Print and shaded views of the part. All mm, measured from the part's lowest x, y and z. A direction names the side the tool comes from. Coordinates: 2 decimals unless noted, no trailing zeros. Write item = value, one per line.
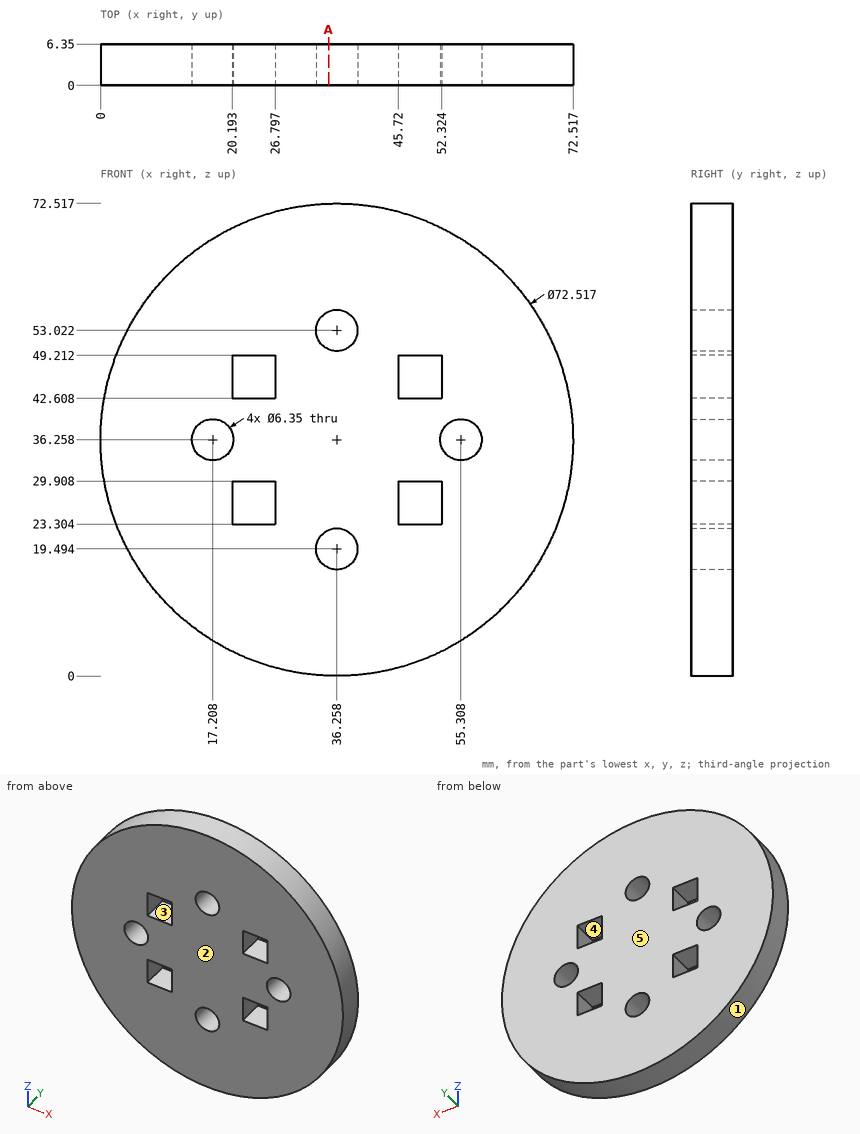
Q1. Probe line 1 (X direction, y = 4, z = 38) (1 decimal); line 2 (X direction, y = 4.75, z = 29) (1 decimal); line 3 (Z direction, x = 39, y = 2.5) (1 decimal). List the from-to ranges inside material, lowest first. Write a range as from..to.
Model answer:
line_1 = 0..14.6, 19.9..52.7, 58..72.5
line_2 = 0.7..20.2, 26.8..45.7, 52.3..71.8
line_3 = 0.1..17.9, 21.1..51.4, 54.6..72.4
Q2. Pin check, flat tips, straight feed: pin 1 (3 mm diameter, centred on y = 4.5, z = 44.5, fed in from +X) (1 decimal); pin 2 (1 mm diameter, centred on y = 2.5, z = 35.5, fed in from -X); pin 3 (3 mm diameter, centred on y = 3, z = 28, fed in from -X) (1 decimal). Stop position of each tip, or through.
Model answer:
pin_1 = 71.9
pin_2 = 0
pin_3 = 0.6
Q3. Which spindle directions (+Z, -Z, +X, -X, +Y, -Y) get a long thin tool onto all of the face, cutting with end or side? Do the marked faces 4 and 5. Say none if no direction does.
Model answer:
face_4 = +Y, -Y
face_5 = +Z, -Z, +X, -X, +Y
Q4. Mould opens along X. For the marked faces 1, 2 and 3 say: released by +X, released by -X, zero draft, split by the parting line, or undercut.
Model answer:
face_1 = split by the parting line
face_2 = zero draft
face_3 = undercut
Q5. Saw through at A-A on x = 35. Count the separate pieces of the cut face and the enclosed holes in it, and give its area (3 significant figures).
Model answer:
separate_pieces = 3
enclosed_holes = 0
area = 386 mm²
